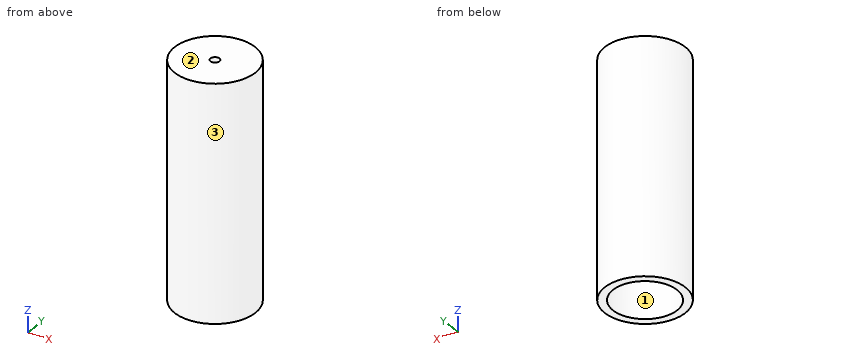
```python
from build123d import *

# Parameters (mm, degrees)
SKETCH2_R           = 22
BOSS_EXTRUDE1_DEPTH = 127.5
SKETCH3_R           = 2.5
CUT_EXTRUDE1_DEPTH  = 135
SKETCH5_R           = 17.5
CUT_EXTRUDE2_DEPTH  = 30


with BuildPart() as part:
    # Sketch2 → Boss-Extrude1 (new body)
    with BuildSketch(Plane.XY):
        Circle(SKETCH2_R)
    extrude(amount=BOSS_EXTRUDE1_DEPTH)

    # Sketch3 → Cut-Extrude1 (cut)
    with BuildSketch(Plane(origin=(0, 0, 0), x_dir=(-1, 0, 0), z_dir=(0, 0, -1))):
        Circle(SKETCH3_R)
    extrude(amount=-CUT_EXTRUDE1_DEPTH, mode=Mode.SUBTRACT)

    # Sketch5 → Cut-Extrude2 (cut)
    with BuildSketch(Plane(origin=(0, 0, 0), x_dir=(-1, 0, 0), z_dir=(0, 0, -1))):
        Circle(SKETCH5_R)
    extrude(amount=-CUT_EXTRUDE2_DEPTH, mode=Mode.SUBTRACT)


solid = part.part
```
The listing builds one solid part. Answer for the finished solid, in the listing's coordinates (mm). Face numbers are marked on the shaded views. Give positions to 0.01 mm unless a question says otherwise; leave off trailing zeros. Order: outer loops, then holes, each group sorted by start corner. A loop starts at its lowest first (then second) coordinate and runs counter-clockwise, first axis right, second up. Notation, with made-up numbers: (-6.75, -28.75) -> (52.25, -28.75) arc R25 ccw to (52.25, -16.75) -> close; hole circle Ø6 at (47.25, -12). An arc over 180 degrees is marked (long way). One line per item, written item: value.
1) Flat-ended cylindrical pins translate along their axes: P1, Ø4.5, axis at x = 0, y = 0, coming from the +Z side; P2, Ø4, axis at x = -11.5, y = 6.5, coming from the -Z side; P3, Ø1, axis at x = 8.5, z = 66, coming from the +Y side; P4, Ø1, axis at x = -16.5, z = 52, coming from the -Y side. Find the tip coordinate at first contact, or state that the pin passes through.
Reported:
P1: passes through
P2: stops at z = 30
P3: stops at y = 20.49
P4: stops at y = -15.1
2) Find section D-D, the plane y = 11. Determine the outline of the cut face in (x, z), plus the area to 3 significant figures.
Reported:
outline: (-19.05, 0) -> (-13.61, 0) -> (-13.61, 30) -> (13.61, 30) -> (13.61, 0) -> (19.05, 0) -> (19.05, 127.5) -> (-19.05, 127.5) -> close
area: 4,040 mm^2
3) Determine the mould class of the marked faces 1, 2 and 3 for opening direction X: pulls with the +X half, pulls with the -X half, needs draft (parallel to the pull), parting line crosses it, or undercut.
Reported:
face 1: undercut
face 2: needs draft
face 3: parting line crosses it
4) Find section C-C, the plane z = 14.5. Determine the outline of the cut face in (x, y), plus the area to 3 significant figures.
Reported:
outline: circle Ø44 at (0, 0); hole circle Ø35 at (0, 0)
area: 558 mm^2
5) Find the intervals of material crossed by line 1 (Y direction, x = 0, z = 76.5); line 2 (Y direction, x = 0, z = 7.75); line 3 (Z direction, x = -3, y = -15), in increasing order.
Reported:
line 1: y = -22 to -2.5, 2.5 to 22
line 2: y = -22 to -17.5, 17.5 to 22
line 3: z = 30 to 127.5
6) Find section A-A, the plane y = 0. Determine the outline of the cut face in (x, z).
Reported:
outline: (-22, 0) -> (-17.5, 0) -> (-17.5, 30) -> (-2.5, 30) -> (-2.5, 127.5) -> (-22, 127.5) -> close; (2.5, 30) -> (17.5, 30) -> (17.5, 0) -> (22, 0) -> (22, 127.5) -> (2.5, 127.5) -> close
